Source: CAD feature listing. Evaluate the final solid. Frame: model axes, mm. Face numbers are marked on the shaded views. A direction names the side the tool comes from. Round coordinates to 2 decimals unless told otherwise and drop trailing zeros. Write each loop counter-clockwise with the first axis right and the second up, starting at its lowest first coordinate (ties: lowest second). Pieces come first, ordered by that corner, then holes. Notation, with made-up numbers: M -1,34.25 L 40,34.25 A33 cw 40,64.25 Z; hole C 89.5,52.5 d7. An arc over 180 degrees is marked long. Answer in a Markdown table with one row per item. Add a question column.
Item 1: Cut plane B-B on z = 11.5. Return loops of the section in (x, y), and give its area (3 significant figures).
Item 2: Contact query for flat-ended pins moving along their axis: pin 1 (1.4 mm diameter, centred on x = 27, z = 18.5, fed in from -Y); pin 2 (0.6 mm diameter, centred on x = 43, y = -99.5, fed in from +Z); pin 3 (12 mm diameter, centred on x = 10.5, y = -26.5, fed in from +Z). Output: stop coordinate, or through.
Item 3: Cut plane C-C on x = 41. Return loops of the section in (y, z), and give its area (3 significant figures).
Item 4: Material intervals for probe 1 along Y at (x, z) = (40.5, 6); probe 2 along X at (y, z) = (-55.5, 2.5); probe 3 along X at (y, z) = (-65, 18.5), sorted ascending.
Item 5: Mould query, pull axis Y, two halves, no side actions, for the marked faces 3, 4 and 5. Classes: released by +Y, released by -Y, zero draft, split by the parting line, or undercut.
Item 6: Set-up query: the marked faces 1 and 2. Return all of +Z, -Z, +X, -X, +Y, -Y with unobstructed straight access to the full face (end or side cutting, diameter ignored); none if empty.
Item 7: Cut plane A-A on y = -40. Return loops of the section in (x, z).
from build123d import *

# Parameters (mm, degrees)
F0_W     = 70
F0_H     = 100
F1_DEPTH = 20
F2_W     = 66
F2_H     = 96
F3_DEPTH = 18
F4_W     = 65.9895728827
F4_H     = 2
F5_DEPTH = 2.5
F7_DEPTH = 98
F8_W     = 66
F8_H     = 1.7997355314
F9_DEPTH = 1


with BuildPart() as f1:
    # F0 (on Top) → F1 (new body)
    with BuildSketch(Plane.XY):
        with Locations((35, -50)):
            Rectangle(F0_W, F0_H)
    extrude(amount=F1_DEPTH)

    # F2 (on face) → F3 (cut)
    with BuildSketch(Plane.XY.offset(20)):
        with Locations((35, -50)):
            Rectangle(F2_W, F2_H)
    extrude(amount=-F3_DEPTH, mode=Mode.SUBTRACT)

    # F4 (on face) → F5 (cut)
    with BuildSketch(Plane.XY.offset(20)):
        with Locations((34.9947864413, -99)):
            Rectangle(F4_W, F4_H)
    extrude(amount=-F5_DEPTH, mode=Mode.SUBTRACT)

    # F6 (on face) → F7 (cut)
    with BuildSketch(Plane.XZ.offset(100)):
        with BuildLine():
            Line((67.9895728827, 19.4992875666), (67.9895728827, 17.5))
            ThreePointArc((67.9895728827, 17.5), (68.7138689095, 17.7831631236), (69.016261954, 18.4996437833))
            ThreePointArc((69.016261954, 18.4996437833), (68.7138689095, 19.216124443), (67.9895728827, 19.4992875666))
        make_face()
        with BuildLine():
            ThreePointArc((2, 19.4998536759), (1.0120962274, 18.499926838), (2, 17.5))
            Line((2, 17.5), (2, 19.4998536759))
        make_face()
    extrude(amount=-F7_DEPTH, mode=Mode.SUBTRACT)

    # F8 (on face) → F9 (cut)
    with BuildSketch(Plane.XZ.offset(2)):
        with Locations((35, 18.4996437833)):
            Rectangle(F8_W, F8_H)
    extrude(amount=-F9_DEPTH, mode=Mode.SUBTRACT)


solid = f1.part
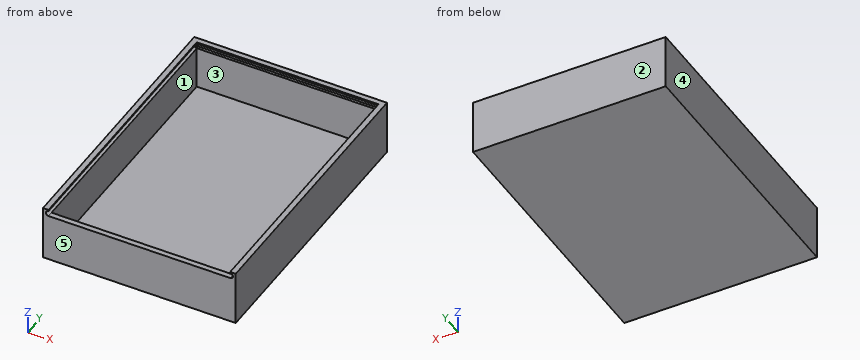
Results below:
| question | item | result |
|---|---|---|
| 1 | outline | M 0,-100 L 70,-100 L 70,0 L 0,0 Z; hole M 2,-98 L 68,-98 L 68,-2 L 2,-2 Z |
| 1 | area | 664 mm2 |
| 2 | pin 1 | y = -1 |
| 2 | pin 2 | z = 17.5 |
| 2 | pin 3 | z = 2 |
| 3 | outline | M -100,0 L 0,0 L 0,20 L -2,20 L -2,19.4 L -1,19.4 L -1,17.6 L -2,17.6 L -2,2 L -98,2 L -98,17.5 L -100,17.5 Z |
| 3 | area | 265 mm2 |
| 4 | probe 1 | -100 to -98, -2 to 0 |
| 4 | probe 2 | 0 to 2, 68 to 70 |
| 4 | probe 3 | 0 to 1.01, 69.02 to 70 |
| 5 | face 3 | undercut |
| 5 | face 4 | zero draft |
| 5 | face 5 | released by -Y |
| 6 | face 1 | +Z |
| 6 | face 2 | +Z, -Z, +X, -X, +Y |
| 7 | outline | M 0,0 L 70,0 L 70,20 L 68,20 L 68,19.5 A1 cw long 68,17.5 L 68,2 L 2,2 L 2,17.5 A1 cw 2,19.5 L 2,20 L 0,20 Z |
